Geometry check sheet. Reference: drawing and pictorial views, mm from the part's lowest x, y, z. A direction names the side the tool comes from. Give positions to 0.01 mm unless a question says otherwise; leave off trailing zeros. Write each loop counter-clockwise with the first axis right and the second up, starting at its lowest first coordinate (ties: lowest second). Pieces come first, ordered by that corner, then holes.
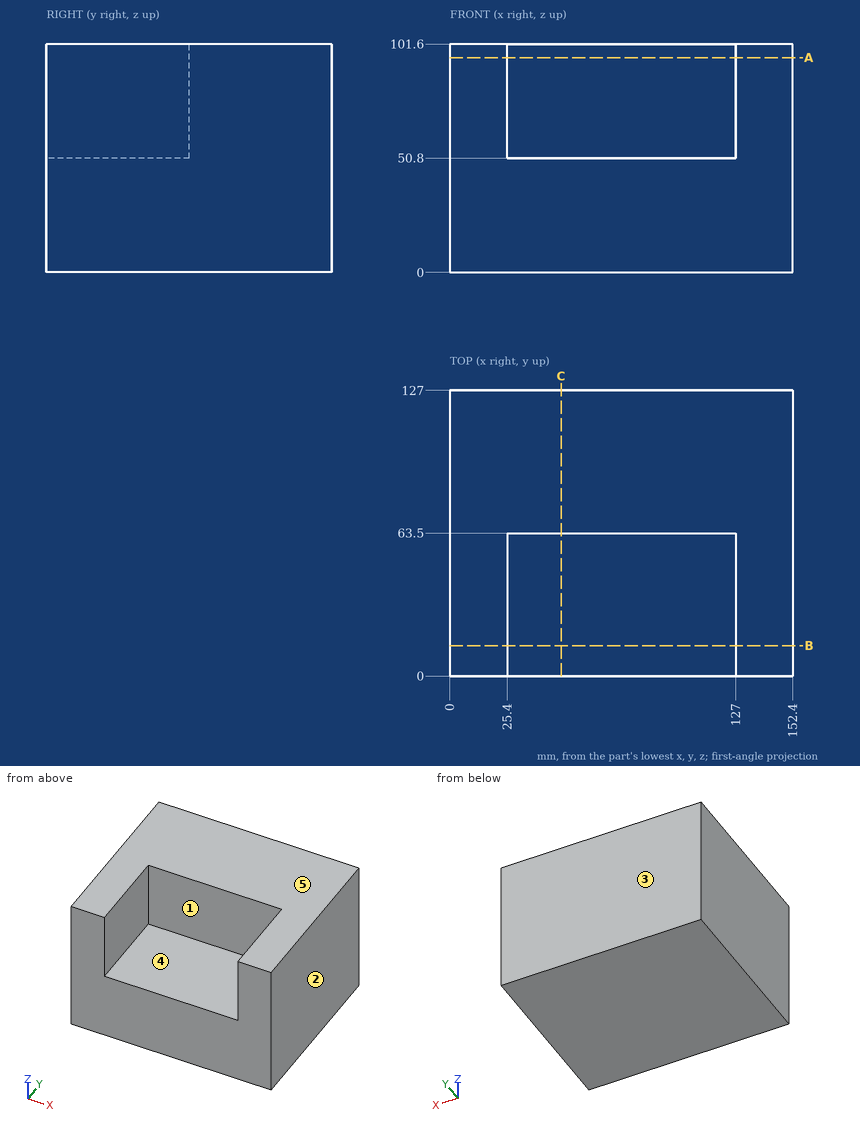
Item 1: Set-up check for the marked faces 4 and 5: record each of +Z, -Z, +X, -X, +Y, -Y from which the full face is reachable in a straight line by a thin tool's end or side.
Answer key:
face 4: +Z, -Y
face 5: +Z, +X, -X, +Y, -Y
Item 2: Release check for a two-part mould opening along X. For the marked faces 1, 2 and 3 record: released by +X, released by -X, zero draft, split by the parting line, or undercut.
Answer key:
face 1: undercut
face 2: released by +X
face 3: zero draft
Item 3: Sectioned sample at C-C on x = 49.5. Record the cut outline in (y, z), then the cut area to 3 significant figures.
Answer key:
outline: (0, 0) - (127, 0) - (127, 101.6) - (63.5, 101.6) - (63.5, 50.8) - (0, 50.8) - close
area: 9,680 mm2
Item 4: Sectioned sample at B-B on y = 13.5. Record the cut outline in (x, z).
Answer key:
outline: (0, 0) - (152.4, 0) - (152.4, 101.6) - (127, 101.6) - (127, 50.8) - (25.4, 50.8) - (25.4, 101.6) - (0, 101.6) - close
Item 5: Sectioned sample at A-A on z = 95.5. Record the cut outline in (x, y).
Answer key:
outline: (0, 0) - (25.4, 0) - (25.4, 63.5) - (127, 63.5) - (127, 0) - (152.4, 0) - (152.4, 127) - (0, 127) - close
Item 6: Scan lines: line 1 along X through (y, z) = (8, 77.5); line 2 along Y through (x, z) = (63, 59); line 3 along Z through (x, y) = (96, 36.5). Record each from-to range of solid material in increasing order.
Answer key:
line 1: x = 0 to 25.4, 127 to 152.4
line 2: y = 63.5 to 127
line 3: z = 0 to 50.8
Item 7: Depth check by flat-ended pin: pin 1 (3 mm diameter, centred on x = 38, z = 58, fed in from -Y); pin 2 (19 mm diameter, centred on x = 87, y = 18.5, fed in from +Z). Enter the tip coordinate at first touch or a pass-through.
Answer key:
pin 1: stops at y = 63.5
pin 2: stops at z = 50.8
